```python
from build123d import *

# Parameters (mm, degrees)
F0_R      = 30.625
F1_DEPTH  = 1.6
F2_W      = 5.6
F2_H      = 5.6
F3_DEPTH  = 2.5
F4_W      = 16
F4_H      = 16
F5_DEPTH  = 1.6
F4_W_2    = 5.6
F4_H_2    = 5.6
F6_DEPTH  = 2.5
F4_W_3    = 3.4
F4_H_3    = 3
F4_W_4    = 1
F4_H_4    = 1.4143656492
F7_DEPTH  = 2.5
F8_DEPTH  = 3.5
F4_W_5    = 19
F4_H_5    = 8
F10_DEPTH = 4.5
F4_W_6    = 4.9
F4_H_6    = 11.6
F11_DEPTH = 0.7
F12_DEPTH = 4.3
F13_DEPTH = 3.5


# Not quite as in the source:
# - the program builds the solid bodies; features that only make, move or delete a surface that nothing else refers to are left out


with BuildPart() as f1:
    # F0 (on Front) → F1 (new body)
    with BuildSketch(Plane.XZ):
        Circle(F0_R)
    extrude(amount=F1_DEPTH)

    # F2 (on face) → F3 (join)
    with BuildSketch(Plane.XZ.offset(1.6)):
        with Locations((-26.67, 0)):
            Rectangle(F2_W, F2_H)
        with Locations((-18.8585378542, 18.8585378542)):
            Rectangle(F2_W, F2_H)
        with Locations((0, 26.67)):
            Rectangle(F2_W, F2_H)
        with Locations((18.8585378542, 18.8585378542)):
            Rectangle(F2_W, F2_H)
        with Locations((26.67, 0)):
            Rectangle(F2_W, F2_H)
        with Locations((18.8585378542, -18.8585378542)):
            Rectangle(F2_W, F2_H)
        with Locations((0, -26.67)):
            Rectangle(F2_W, F2_H)
        with Locations((-18.8585378542, -18.8585378542)):
            Rectangle(F2_W, F2_H)
    extrude(amount=F3_DEPTH)

    # F4 (on face) → F5 (join)
    with BuildSketch(Plane(origin=(0, 0, 0), x_dir=(-1, 0, 0), z_dir=(0, 1, 0))):
        with Locations((-9, -7)):
            Rectangle(F4_W, F4_H)
    extrude(amount=F5_DEPTH)

    # F4 (on face) → F6 (join)
    with BuildSketch(Plane(origin=(0, 0, 0), x_dir=(-1, 0, 0), z_dir=(0, 1, 0))):
        with Locations((0, 25)):
            Rectangle(F4_W_2, F4_H_2)
    extrude(amount=F6_DEPTH)

    # F4 (on face) → F7 (join)
    with BuildSketch(Plane(origin=(0, 0, 0), x_dir=(-1, 0, 0), z_dir=(0, 1, 0))):
        with Locations((7, 24)):
            Rectangle(F4_W_3, F4_H_3)
        with Locations((7, 24)):
            Rectangle(F4_W_4, F4_H_4, mode=Mode.SUBTRACT)
    extrude(amount=F7_DEPTH)

    # F4 (on face) → F8 (join)
    with BuildSketch(Plane(origin=(0, 0, 0), x_dir=(-1, 0, 0), z_dir=(0, 1, 0))):
        with Locations((7, 24)):
            Rectangle(F4_W_4, F4_H_4)
    extrude(amount=F8_DEPTH)

    # F4 (on face) → F10 (join)
    with BuildSketch(Plane(origin=(0, 0, 0), x_dir=(-1, 0, 0), z_dir=(0, 1, 0))):
        with Locations((0, -22.225)):
            Rectangle(F4_W_5, F4_H_5)
    extrude(amount=F10_DEPTH)

    # F4 (on face) → F11 (join)
    with BuildSketch(Plane(origin=(0, 0, 0), x_dir=(-1, 0, 0), z_dir=(0, 1, 0))):
        with Locations((-25, -5)):
            Rectangle(F4_W_6, F4_H_6)
        with BuildLine():
            ThreePointArc((-26.9, -1.75), (-25, 0.15), (-23.1, -1.75))
            Line((-23.1, -1.75), (-23.1, -8.25))
            ThreePointArc((-23.1, -8.25), (-25, -10.15), (-26.9, -8.25))
            Line((-26.9, -8.25), (-26.9, -1.75))
        make_face(mode=Mode.SUBTRACT)
    extrude(amount=F11_DEPTH)

    # F4 (on face) → F12 (join)
    with BuildSketch(Plane(origin=(0, 0, 0), x_dir=(-1, 0, 0), z_dir=(0, 1, 0))):
        with BuildLine():
            Line((-23.1, -8.25), (-23.1, -1.75))
            ThreePointArc((-23.1, -1.75), (-25, 0.15), (-26.9, -1.75))
            Line((-26.9, -1.75), (-26.9, -8.25))
            ThreePointArc((-26.9, -8.25), (-25, -10.15), (-23.1, -8.25))
        make_face()
    extrude(amount=F12_DEPTH)

    # F4 (on face) → F13 (join)
    with BuildSketch(Plane(origin=(0, 0, 0), x_dir=(-1, 0, 0), z_dir=(0, 1, 0))):
        with BuildLine():
            Line((24.005, -3.81), (30.387078257, -3.81))
            ThreePointArc((30.387078257, -3.81), (30.5654616898, -1.90871074), (30.625, 0))
            ThreePointArc((30.625, 0), (30.5654616898, 1.90871074), (30.387078257, 3.81))
            Line((30.387078257, 3.81), (24.005, 3.81))
            Line((24.005, 3.81), (24.005, -3.81))
        make_face()
        with BuildLine():
            Line((30.387078257, -3.81), (31.625, -3.81))
            Line((31.625, -3.81), (31.625, 3.81))
            Line((31.625, 3.81), (30.387078257, 3.81))
            ThreePointArc((30.387078257, 3.81), (30.5654616898, 1.90871074), (30.625, 0))
            ThreePointArc((30.625, 0), (30.5654616898, -1.90871074), (30.387078257, -3.81))
        make_face()
    extrude(amount=F13_DEPTH)


solid = f1.part
```
Work out the finished part from the listing and answer in its coordinate system (mm). A direction names the side the tool comes from. Coordinates: 2 decimals unless noted, no trailing zeros. Loops run counter-clockwise (first coordinate to the right, second up) from the corner with the lowest first, then second, coordinate; pieces in that order, holes last.
1) Section A-A (x = 0) is taken. Give the vertices of the cut face in (y, z) (3 decimals).
Results:
outline: (-4.1, -29.47) - (-1.6, -29.47) - (-1.6, -30.625) - (0, -30.625) - (0, -26.225) - (4.5, -26.225) - (4.5, -18.225) - (0, -18.225) - (0, 22.2) - (2.5, 22.2) - (2.5, 27.8) - (0, 27.8) - (0, 30.625) - (-1.6, 30.625) - (-1.6, 29.47) - (-4.1, 29.47) - (-4.1, 23.87) - (-1.6, 23.87) - (-1.6, -23.87) - (-4.1, -23.87) - close
2) Section B-B (z = -19.5) is taken. Give the vertices of the cut face in (x, y).
Results:
outline: (-23.61, -1.6) - (-21.66, -1.6) - (-21.66, -4.1) - (-16.06, -4.1) - (-16.06, -1.6) - (16.06, -1.6) - (16.06, -4.1) - (21.66, -4.1) - (21.66, -1.6) - (23.61, -1.6) - (23.61, 0) - (9.5, 0) - (9.5, 4.5) - (-9.5, 4.5) - (-9.5, 0) - (-23.61, 0) - close
3) Consider probe 1 along X at (y, z) = (-2.75, 17.5); probe 2 along Z at (x, y) = (-6.5, 0.5) (3 decimals). Determine where each line is inside the solid, lowest interval first.
Results:
probe 1: x = -21.66 to -16.06, 16.06 to 21.66
probe 2: z = -26.225 to -18.225, 22.5 to 25.5
4) For a pull along Z with two mould halves and no side action, classify faces 1 (the flat face through (-24.005, 2, 0)), 2 (the flat face through (-7, 1, 25.5)), 3 (the flat face through (0, -1.6, 0)) as +Z half, -Z half, draft (parallel to the pull), parting line (faces both ways), or undercut.
Results:
face 1: draft
face 2: +Z half
face 3: undercut
5) Section D-D (z = 26.5) is taken. Give the vertices of the cut face in (x, y), plus the area to 3 significant figures.
Results:
outline: (-15.35, -1.6) - (-2.8, -1.6) - (-2.8, -4.1) - (2.8, -4.1) - (2.8, -1.6) - (15.35, -1.6) - (15.35, 0) - (2.8, 0) - (2.8, 2.5) - (-2.8, 2.5) - (-2.8, 0) - (-15.35, 0) - close
area: 77.1 mm2
6) Flat-ended cylindrical pins translate along their axes: pin 1 (0.8 mm diameter, centred on x = 0.5, y = 1.5, fed in from -Z) (3 decimals); pin 2 (0.7 mm diameter, centred on y = -3, z = 0.5, fed in from -X); pin 3 (0.8 mm diameter, centred on y = 1, z = 24, fed in from +X). Find the tip coordinate at first contact, or state that the pin passes through.
Results:
pin 1: stops at z = -26.225
pin 2: stops at x = -29.47
pin 3: stops at x = 2.8
7) For faces 4 (the flat face through (-8.7, 1, 24)), 5 (the flat face through (9, 1, -15)), 6 (the flat face through (-23.87, -3, 0)), 7 (the flat face through (-28, 3.5, 0)), 8 (the flat face through (21.659, -3, 19)), determine the directions among +Z, -Z, +X, -X, +Y, -Y from which every point of the face is accessible in a straight line to the end or side of a thin tool.
Results:
face 4: +Z, -X, +Y
face 5: +X, -X, +Y
face 6: +Z, -Z, -Y
face 7: +Z, -Z, -X, +Y
face 8: +Z, -Z, +X, -Y
8) Section C-C (x = 7) is taken. Give the vertices of the cut face in (y, z) (3 decimals), plus the area to 3 significant figures.
Results:
outline: (-1.6, -29.814) - (0, -29.814) - (0, -26.225) - (4.5, -26.225) - (4.5, -18.225) - (0, -18.225) - (0, -15) - (1.6, -15) - (1.6, 1) - (0, 1) - (0, 29.814) - (-1.6, 29.814) - close
area: 157 mm2
